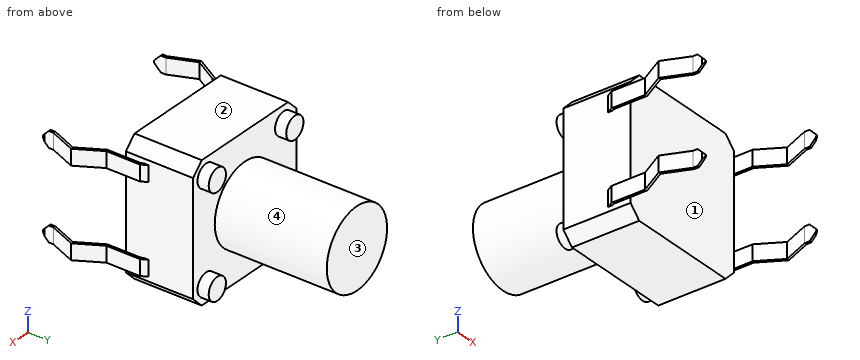
```python
from build123d import *

# Parameters (mm, degrees)
SKETCH1_W               = 6.01
SKETCH1_H               = 6.01
BOSS_EXTRUDE1_DEPTH     = 3
CHAMFER1_SIZE           = 0.5
SKETCH3_R               = 1.75
BOSS_EXTRUDE2_DEPTH     = 5
SKETCH4_R               = 0.5
BOSS_EXTRUDE6_DEPTH     = 0.5
SKETCH5_R               = 0.5
BOSS_EXTRUDE7_DEPTH     = 0.5
SKETCH6_W               = 0.7
SKETCH6_H               = 0.2
MIRROR2_COPY_1_SKETCH_W = 0.7
MIRROR2_COPY_1_SKETCH_H = 0.2
CUT_EXTRUDE1_DEPTH      = 4.782799277


with BuildPart() as part:
    # Sketch1 → Boss-Extrude1 (new body)
    with BuildSketch(Plane(origin=(0, 0, 0), x_dir=(1, 0, 0), z_dir=(0, 1, 0))):
        Rectangle(SKETCH1_W, SKETCH1_H)
    extrude(amount=BOSS_EXTRUDE1_DEPTH)

    # Chamfer1
    chamfer1_edges = [part.edges().sort_by_distance(p)[0] for p in [
        (3.005, 1.5, 3.005),
        (-3.005, 1.5, 3.005),
        (-3.005, 1.5, -3.005),
        (3.005, 1.5, -3.005),
    ]]
    chamfer(chamfer1_edges, length=CHAMFER1_SIZE)

    # Sketch3 → Boss-Extrude2 (add)
    with BuildSketch(Plane(origin=(0, 3, 0), x_dir=(1, 0, 0), z_dir=(0, 1, 0))):
        Circle(SKETCH3_R)
    extrude(amount=BOSS_EXTRUDE2_DEPTH)

    # Sketch4 → Boss-Extrude6 (add)
    with BuildSketch(Plane(origin=(0, 3, 0), x_dir=(1, 0, 0), z_dir=(0, 1, 0))):
        with Locations((2.25, 2.25)):
            Circle(SKETCH4_R)
        with Locations((2.25, -2.25)):
            Circle(SKETCH4_R)
        with Locations((-2.25, 2.25)):
            Circle(SKETCH4_R)
    extrude(amount=BOSS_EXTRUDE6_DEPTH)

    # Sketch5 → Boss-Extrude7 (add)
    with BuildSketch(Plane(origin=(0, 3, 0), x_dir=(1, 0, 0), z_dir=(0, 1, 0))):
        with Locations((-2.25, -2.25)):
            Circle(SKETCH5_R)
    extrude(amount=BOSS_EXTRUDE7_DEPTH)

    # Sweep1: sweep along a path in Sketch7
    with BuildLine(Plane.XY) as sweep1_path:
        Line((-3.005, 0.9), (-3.105, 0.726794919))
        Line((-3.105, 0.726794919), (-3.105, -0.773205081))
        Line((-3.105, -0.773205081), (-3.72715614, -1.850811126))
        Line((-3.72715614, -1.850811126), (-3.25, -3))
        Line((-3.25, -3), (-3.25, -3.5))
    # Sketch6 → Sweep1 (sweep)
    with BuildSketch(Plane.ZY.offset(3.005)):
        with Locations((-1.955, 0.9)):
            Rectangle(SKETCH6_W, SKETCH6_H)
    sweep1 = sweep(path=sweep1_path.line, transition=Transition.RIGHT)

    # Mirror1: Sweep1 across plane
    add(sweep1.mirror(Plane.XY))

    # Mirror2: Sweep1 across plane
    add(sweep1.mirror(Plane(origin=(0, 0, 0), x_dir=(0, 0, 1), z_dir=(1, 0, 0))))

    # Mirror2 copy 1: sweep along a path in Mirror2 copy 1 path
    with BuildLine(Plane(origin=(0, 0, 0), x_dir=(-1, 0, 0), z_dir=(0, 0, -1))) as mirror2_copy_1_path:
        Line((-3.005, 0.9), (-3.105, 0.726794919))
        Line((-3.105, 0.726794919), (-3.105, -0.773205081))
        Line((-3.105, -0.773205081), (-3.72715614, -1.850811126))
        Line((-3.72715614, -1.850811126), (-3.25, -3))
        Line((-3.25, -3), (-3.25, -3.5))
    # Mirror2 copy 1 sketch → Mirror2 copy 1 (sweep)
    with BuildSketch(Plane(origin=(3.005, 0, 0), x_dir=(0, 0, -1), z_dir=(1, 0, 0))):
        with Locations((-1.955, 0.9)):
            Rectangle(MIRROR2_COPY_1_SKETCH_W, MIRROR2_COPY_1_SKETCH_H)
    sweep(path=mirror2_copy_1_path.line, transition=Transition.RIGHT)

    # Sketch8 → Cut-Extrude1 (cut, symmetric)
    with BuildSketch(Plane(origin=(0, 0, 0), x_dir=(0, 0, -1), z_dir=(1, 0, 0))):
        with BuildLine():
            Line((-2.305, -3.211682602), (-2.305, -3.58660254))
            Line((-2.305, -3.58660254), (-1.605, -3.58660254))
            Line((-1.605, -3.58660254), (-1.605, -3.211682602))
            Line((-1.605, -3.211682602), (-1.881694927, -3.48928466))
            ThreePointArc((-1.881694927, -3.48928466), (-1.952077784, -3.518688814), (-2.022718654, -3.489910032))
            Line((-2.022718654, -3.489910032), (-2.305, -3.211682602))
        make_face()
    cut_extrude1 = extrude(amount=CUT_EXTRUDE1_DEPTH, both=True, mode=Mode.SUBTRACT)

    # Mirror3: Cut-Extrude1 across plane
    add(cut_extrude1.mirror(Plane.XY), mode=Mode.SUBTRACT)


solid = part.part
```
Work out the finished part from the listing and answer in its coordinate system (mm). Face numbers are marked on the shaded views. A direction names the side the tool comes from. Coordinates: 2 decimals unless noted, no trailing zeros. Loops run counter-clockwise (first coordinate to the right, second up) from the corner with the lowest first, then second, coordinate; pieces in that order, holes last. Notation, with made-up numbers: (23, 62.5) - (81, 62.5) arc R12 ccw to (81, 72.5) - close; hole circle Ø5 at (15.5, 50). An arc over 180 degrees is marked (long way). Use a Markdown table: item, result.
Item 1: Given pin 1 Ø1 at (x, z) = (2, -0.5) entering from -Y; pin 2 Ø0.8 at (x, z) = (-2, -2.5) entering from +Y; pin 3 Ø0.6 at (y, z) = (-3, -2) entering from -X; pin 4 Ø2 at (y, z) = (-2, -0.5) entering from -X, each flat-ended and moving along its own axis, determine where each tip first touches the part or whether it passes through.
Evaluation:
| item | result |
|---|---|
| pin 1 | stops at y = 0 |
| pin 2 | stops at y = 3.5 |
| pin 3 | stops at x = -3.43 |
| pin 4 | passes through |
Item 2: Find section D-D, the plane x = 2.25. Determine the outline of the cut face in (y, z) (3 decimals), and give its area (3 significant figures).
Evaluation:
| item | result |
|---|---|
| outline | (0, -3.005) - (3, -3.005) - (3, -2.75) - (3.5, -2.75) - (3.5, -1.75) - (3, -1.75) - (3, 1.75) - (3.5, 1.75) - (3.5, 2.75) - (3, 2.75) - (3, 3.005) - (0, 3.005) - close |
| area | 19.0 mm2 |
Item 3: Find section A-A, the plane y = -0.5. Determine the outline of the cut face in (x, z) (3 decimals).
Evaluation:
| item | result |
|---|---|
| outline | (-3.155, -2.305) - (-3.055, -2.305) - (-3.055, -1.605) - (-3.155, -1.605) - close; (-3.155, 1.605) - (-3.055, 1.605) - (-3.055, 2.305) - (-3.155, 2.305) - close; (3.055, -2.305) - (3.155, -2.305) - (3.155, -1.605) - (3.055, -1.605) - close; (3.055, 1.605) - (3.155, 1.605) - (3.155, 2.305) - (3.055, 2.305) - close |
Item 4: The mould has two halves that part along X. Classify the marked faces 1 and 2: +X half, -X half, draft (parallel to the pull), parting line (faces both ways), or undercut.
Evaluation:
| item | result |
|---|---|
| face 1 | undercut |
| face 2 | draft |
Item 5: For the marked faces 3 and 4, determine the directions among +Z, -Z, +X, -X, +Y, -Y from which every point of the face is accessible in a straight line to the end or side of a thin tool.
Evaluation:
| item | result |
|---|---|
| face 3 | +Z, -Z, +X, -X, +Y |
| face 4 | +Y |
Item 6: Find section B-B, the plane z = 0. Determine the outline of the cut face in (x, y) (3 decimals), and give its area (3 significant figures).
Evaluation:
| item | result |
|---|---|
| outline | (-3.005, 0) - (3.005, 0) - (3.005, 3) - (1.75, 3) - (1.75, 8) - (-1.75, 8) - (-1.75, 3) - (-3.005, 3) - close |
| area | 35.5 mm2 |
Item 7: Consider probe 1 along X at (y, z) = (2.5, 0) (3 decimals); probe 2 along Y at (x, z) = (-0.25, 2.5); probe 3 along Y at (x, z) = (-0.75, -1). Determine where each line is inside the solid, lowest interval first. Write a range as from..to.
Evaluation:
| item | result |
|---|---|
| probe 1 | x = -3.005..3.005 |
| probe 2 | y = 0..3 |
| probe 3 | y = 0..8 |
Item 8: Find section C-C, the plane x = 0. Determine the outline of the cut face in (y, z) (3 decimals).
Evaluation:
| item | result |
|---|---|
| outline | (0, -3.005) - (3, -3.005) - (3, -1.75) - (8, -1.75) - (8, 1.75) - (3, 1.75) - (3, 3.005) - (0, 3.005) - close |
